Model file for the job. Use its own axes, mm. A direction names the side the tool comes from. Coordinates: 2 decimals unless noted, no trailing zeros. Write each loop counter-clockwise with the first axis right and the second up, starting at its lowest first coordinate (ties: lowest second). Pieces come first, ordered by that corner, then holes. Notation, with made-up numbers: M -7.75,18.25 L 0.25,18.25 A13 cw 0.25,41.25 Z; hole C 36.25,20.25 d11. An arc over 180 degrees is marked long. Put each result on its own line as item: value. Start each with the question number.
Q1. Which spindle directions (+Z, -Z, +X, -X, +Y, -Y) get a long thin tool onto all of the face, cutting with end or side? Do faces 1 (the flat face through (-21.844, -18.339, 2.958)), 2 (the flat face through (-21.03, -16.08, 2.96)), 3 (the flat face through (15.684, -12.266, 2.958)). Say none if no direction does.
Q2. Cut at C-C (y = 0). Write the cut outline in (x, z), then the cut area to 3 significant figures.
Q3. Pull direction X, two halves, no side cores. Call faces 4 (the flat face through (16.87, -14.07, 2.96)), 5 (the flat face through (21.656, -18.661, 2.958)), 6 (the flat face through (0, -30, 3)): pulls with the +X half, pulls with the -X half, needs draft (parallel to the pull), parting line crosses it, or undercut.
Q4. Drop flat-ended pins along their axis: pin 1 (8 mm diameter, centred on x = -7.5, y = -15, fed in from -Z); pin 2 (1 mm diameter, centred on y = -12, z = 4.5, fed in from +X); pin 3 (2.5 mm diameter, centred on x = -14.5, z = 4, fed in from +Y); pin 4 (3 mm diameter, centred on x = 14.5, z = 3.5, fed in from +Y). Give the stop position or say it passes through.
Q5. Drill centre lines: line 1 along Z through (x, y) = (5, -29.45); line 2 along X through (y, z) = (-15.5, 0.9); line 3 along Y through (x, z) = (28.5, 1.45). Where is each one in solid material? Low to high.
Q6. Cut at B-B (y = -19). Write the cut outline in (x, z).
Q7. Cut at D-D (x = 25). Write the cut outline in (y, z).
Q8. Cut at A-A (x = -5). Write the cut outline in (y, z).
```python
from build123d import *

# Parameters (mm, degrees)
F1_DEPTH = 6
F2_R     = 1.65
F3_DEPTH = 25


with BuildPart() as f1:
    # F0 (on Top) → F1 (new body)
    with BuildSketch(Plane.XY):
        with BuildLine():
            ThreePointArc((-32, 6.062178), (-32.366025, 4.696152), (-31, 4.330127))
            ThreePointArc((-31, 4.330127), (-23.519027, 0.435779), (-30.210101, -4.698463))
            ThreePointArc((-30.210101, -4.698463), (-31.491813, -5.296136), (-30.894141, -6.577848))
            ThreePointArc((-30.894141, -6.577848), (-29.715537, -6.893654), (-28.5, -7))
            Line((-28.5, -7), (-15, -30))
            Line((-15, -30), (0, -30))
            Line((0, -30), (15, -30))
            Line((15, -30), (28.5, -7))
            ThreePointArc((28.5, -7), (29.715537, -6.893654), (30.894141, -6.577848))
            ThreePointArc((30.894141, -6.577848), (31.491813, -5.296136), (30.210101, -4.698463))
            ThreePointArc((30.210101, -4.698463), (23.519027, 0.435779), (31, 4.330127))
            ThreePointArc((31, 4.330127), (32.366025, 4.696152), (32, 6.062178))
            ThreePointArc((32, 6.062178), (26.279799, 6.638577), (22.057234, 2.736926))
            Line((22.057234, 2.736926), (9.129356, -27.695495))
            ThreePointArc((9.129356, -27.695495), (8.945068, -27.916982), (8.669158, -28))
            Line((8.669158, -28), (0, -28))
            Line((0, -28), (-8.669158, -28))
            ThreePointArc((-8.669158, -28), (-8.945068, -27.916982), (-9.129356, -27.695495))
            Line((-9.129356, -27.695495), (-22.057234, 2.736926))
            ThreePointArc((-22.057234, 2.736926), (-26.279799, 6.638577), (-32, 6.062178))
        make_face()
        with BuildLine():
            Line((-16.143448, -24.745536), (-26.051811, -7.168974))
            ThreePointArc((-26.051811, -7.168974), (-26.089044, -6.760752), (-25.808501, -6.461875))
            ThreePointArc((-25.808501, -6.461875), (-23.883692, -5.262101), (-22.443534, -3.509875))
            ThreePointArc((-22.443534, -3.509875), (-21.984425, -3.261283), (-21.554214, -3.557084))
            Line((-21.554214, -3.557084), (-12.313453, -24.296503))
            ThreePointArc((-12.313453, -24.296503), (-12.350796, -24.772261), (-12.770169, -25))
            Line((-12.770169, -25), (-15.707888, -25))
            ThreePointArc((-15.707888, -25), (-15.960111, -24.931722), (-16.143448, -24.745536))
        make_face(mode=Mode.SUBTRACT)
        with BuildLine():
            ThreePointArc((21.554214, -3.557084), (21.984425, -3.261283), (22.443534, -3.509875))
            ThreePointArc((22.443534, -3.509875), (23.883692, -5.262101), (25.808501, -6.461875))
            ThreePointArc((25.808501, -6.461875), (26.089044, -6.760752), (26.051811, -7.168974))
            Line((26.051811, -7.168974), (16.143448, -24.745536))
            ThreePointArc((16.143448, -24.745536), (15.960111, -24.931722), (15.707888, -25))
            Line((15.707888, -25), (12.770169, -25))
            ThreePointArc((12.770169, -25), (12.350796, -24.772261), (12.313453, -24.296503))
            Line((12.313453, -24.296503), (21.554214, -3.557084))
        make_face(mode=Mode.SUBTRACT)
    extrude(amount=F1_DEPTH)

    # F2 (on face) → F3 (cut)
    with BuildSketch(Plane.XZ.offset(30)):
        with Locations((-5, 3)):
            Circle(F2_R)
        with Locations((5, 3)):
            Circle(F2_R)
    extrude(amount=-F3_DEPTH, mode=Mode.SUBTRACT)


solid = f1.part
```
Computed values:
1. face 1: +Z, -Z, -X, -Y
1. face 2: +Z, -Z
1. face 3: +Z, -Z, +Y
2. outline: M -23.5,0 L -20.89,0 L -20.89,6 L -23.5,6 Z; M 20.89,0 L 23.5,0 L 23.5,6 L 20.89,6 Z
2. area: 31.3 mm2
3. face 4: undercut
3. face 5: pulls with the +X half
3. face 6: needs draft
4. pin 1: through
4. pin 2: x = 25.86
4. pin 3: y = -12.11
4. pin 4: y = -11.52
5. line 1: 0 to 1.35, 4.65 to 6
5. line 2: -23.51 to -21.36, -16.23 to -14.31, 14.31 to 16.23, 21.36 to 23.51
5. line 3: -7 to -5, 5 to 7
6. outline: M -21.46,0 L -19.38,0 L -19.38,6 L -21.46,6 Z; M -14.67,0 L -12.82,0 L -12.82,6 L -14.67,6 Z; M 12.82,0 L 14.67,0 L 14.67,6 L 12.82,6 Z; M 19.38,0 L 21.46,0 L 21.46,6 L 19.38,6 Z
7. outline: M -12.96,0 L -9.03,0 L -9.03,6 L -12.96,6 Z; M -6.06,0 L -3.57,0 L -3.57,6 L -6.06,6 Z; M 3.57,0 L 6.06,0 L 6.06,6 L 3.57,6 Z
8. outline: M -30,0 L -28,0 L -28,1.35 L -30,1.35 Z; M -30,4.65 L -28,4.65 L -28,6 L -30,6 Z
